Check sheet for the modelled part. Datum: model origin and axes. Units: mm. Coordinates: 2 decimals unless noted, no trailing zeros. Loops run counter-clockwise (first coordinate to the right, second up) from the corner with the lowest first, then second, coordinate; pieces in that order, holes last.
from build123d import *

# Parameters (mm, degrees)
SKETCH_R              = 23
SKETCH_R_2            = 2.75
SKETCH_R_3            = 2
PAD_DEPTH             = 1
SKETCH001_R           = 1.65
POCKET_DEPTH          = 1415.215977
POLARPATTERN_COUNT    = 3
POCKET001_DEPTH       = 5
SKETCH003_R           = 1.1
SKETCH003_R_2         = 1.45
POCKET002_DEPTH       = 1.001
SKETCH004_R           = 1.45
POCKET003_DEPTH       = 1.001
SKETCH005_R           = 2.1
POCKET004_DEPTH       = 1.001
SKETCH006_R           = 1.65
POCKET005_DEPTH       = 1415.215977
POLARPATTERN001_COUNT = 4
FILLET_R              = 15
PAD001_DEPTH          = 1


with BuildPart() as part:
    # Sketch → Pad (new body)
    with BuildSketch(Plane.XY):
        Polygon((103.553391, 250), (-103.553391, 250), (-250, 103.553391), (-250, -103.553391), (-103.553391, -250), (103.553391, -250), (250, -103.553391), (250, 103.553391), align=None)
        Circle(SKETCH_R, mode=Mode.SUBTRACT)
        with Locations((150, 150)):
            Circle(SKETCH_R_2, mode=Mode.SUBTRACT)
        with Locations((-150, 150)):
            Circle(SKETCH_R_2, mode=Mode.SUBTRACT)
        with Locations((-150, -150)):
            Circle(SKETCH_R_2, mode=Mode.SUBTRACT)
        with Locations((150, -150)):
            Circle(SKETCH_R_2, mode=Mode.SUBTRACT)
        with Locations((28.284271, 28.284271)):
            Circle(SKETCH_R_3, mode=Mode.SUBTRACT)
        with Locations((-28.284271, 28.284271)):
            Circle(SKETCH_R_3, mode=Mode.SUBTRACT)
        with Locations((-28.284271, -28.284271)):
            Circle(SKETCH_R_3, mode=Mode.SUBTRACT)
        with Locations((28.284271, -28.284271)):
            Circle(SKETCH_R_3, mode=Mode.SUBTRACT)
    extrude(amount=PAD_DEPTH)

    # Sketch001 → Pocket (cut, through all)
    with BuildSketch(Plane.XY):
        with Locations((169.926455, -5)):
            Circle(SKETCH001_R)
        with Locations((169.926455, -18)):
            Circle(SKETCH001_R)
    pocket = extrude(amount=POCKET_DEPTH, mode=Mode.SUBTRACT)

    # PolarPattern: Pocket ×3 about axis
    polarpattern_axis = Axis((0, 0, 0), (0, 0, 1))
    for i in range(1, POLARPATTERN_COUNT):
        add(pocket.rotate(polarpattern_axis, i * 360 / POLARPATTERN_COUNT), mode=Mode.SUBTRACT)

    # Sketch002 → Pocket001 (cut)
    with BuildSketch(Plane.XY):
        with BuildLine():
            ThreePointArc((-60, 8), (-68, 0), (-60, -8))
            Line((-60, -8), (60, -8))
            ThreePointArc((60, -8), (68, 0), (60, 8))
            Line((-60, 8), (60, 8))
        make_face()
    extrude(amount=POCKET001_DEPTH, mode=Mode.SUBTRACT)

    # Sketch003 → Pocket002 (cut, through all)
    with BuildSketch(Plane.XY):
        with Locations((-80, 71)):
            Circle(SKETCH003_R)
        with Locations((-80, 26)):
            Circle(SKETCH003_R)
        with Locations((-80, -26)):
            Circle(SKETCH003_R)
        with Locations((-80, -71)):
            Circle(SKETCH003_R)
        with Locations((-80, 0)):
            Circle(SKETCH003_R_2)
        with Locations((80, 71)):
            Circle(SKETCH003_R)
        with Locations((80, 26)):
            Circle(SKETCH003_R)
        with Locations((80, 0)):
            Circle(SKETCH003_R_2)
        with Locations((80, -26)):
            Circle(SKETCH003_R)
        with Locations((80, -71)):
            Circle(SKETCH003_R)
        Polygon((-95, 51), (-105, 51), (-105, 45), (-103.5, 45), (-103.5, 49.5), (-95, 49.5), align=None)
        Polygon((-105, -45), (-95, -45), (-101.312029, -49.5), (-96, -49.5), (-96, -51), (-106, -51), (-99.687971, -46.5), (-105, -46.5), align=None)
        Polygon((105, -51), (95, -51), (101.312029, -46.5), (96, -46.5), (96, -45), (106, -45), (99.687971, -49.5), (105, -49.5), align=None)
        Polygon((95, 45), (105, 45), (105, 51), (103.5, 51), (103.5, 46.5), (95, 46.5), align=None)
    extrude(amount=POCKET002_DEPTH, mode=Mode.SUBTRACT)

    # Sketch004 → Pocket003 (cut, through all)
    with BuildSketch(Plane.XY):
        with Locations((-32.5, -56.291651)):
            Circle(SKETCH004_R)
        with Locations((32.5, -56.291651)):
            Circle(SKETCH004_R)
        with Locations((-32.5, 56.291651)):
            Circle(SKETCH004_R)
        with Locations((32.5, 56.291651)):
            Circle(SKETCH004_R)
    extrude(amount=POCKET003_DEPTH, mode=Mode.SUBTRACT)

    # Sketch005 → Pocket004 (cut, through all)
    with BuildSketch(Plane.XY):
        with Locations((135, 150)):
            Circle(SKETCH005_R)
        with Locations((165, 150)):
            Circle(SKETCH005_R)
        with Locations((-165, 150)):
            Circle(SKETCH005_R)
        with Locations((-135, 150)):
            Circle(SKETCH005_R)
        with Locations((-165, -150)):
            Circle(SKETCH005_R)
        with Locations((-135, -150)):
            Circle(SKETCH005_R)
        with Locations((135, -150)):
            Circle(SKETCH005_R)
        with Locations((165, -150)):
            Circle(SKETCH005_R)
    extrude(amount=POCKET004_DEPTH, mode=Mode.SUBTRACT)

    # Sketch006 → Pocket005 (cut, through all)
    with BuildSketch(Plane.XY):
        with Locations((-161.970876, -52.035422)):
            Circle(SKETCH006_R)
        with Locations((-157.524615, -64.251426)):
            Circle(SKETCH006_R)
    pocket005 = extrude(amount=POCKET005_DEPTH, mode=Mode.SUBTRACT)

    # PolarPattern001: Pocket005 ×4 about axis
    polarpattern001_axis = Axis((0, 0, 0), (0, 0, 1))
    for i in range(1, POLARPATTERN001_COUNT):
        add(pocket005.rotate(polarpattern001_axis, i * 360 / POLARPATTERN001_COUNT), mode=Mode.SUBTRACT)

    # Fillet
    fillet_edges = [part.edges().sort_by_distance(p)[0] for p in [
        (-250, -103.553391, 0.5),
        (-103.553391, -250, 0.5),
        (103.553391, -250, 0.5),
        (-250, 103.553391, 0.5),
        (-103.553391, 250, 0.5),
        (103.553391, 250, 0.5),
        (250, 103.553391, 0.5),
        (250, -103.553391, 0.5),
    ]]
    fillet(fillet_edges, radius=FILLET_R)

    # Sketch007 → Pad001 (join)
    with BuildSketch(Plane.XY):
        Polygon((369.551813, 153.073373), (153.073373, 369.551813), (-153.073373, 369.551813), (-369.551813, 153.073373), (-369.551813, -153.073373), (-153.073373, -369.551813), (153.073373, -369.551813), (369.551813, -153.073373), align=None)
        Polygon((241.421356, 100), (100, 241.421356), (-100, 241.421356), (-241.421356, 100), (-241.421356, -100), (-100, -241.421356), (100, -241.421356), (241.421356, -100), align=None, mode=Mode.SUBTRACT)
    extrude(amount=PAD001_DEPTH)


solid = part.part
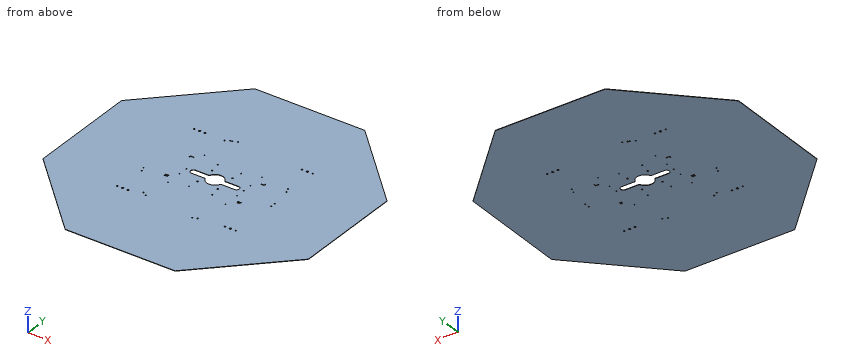
(1) Section check A-A, the plane z = 0.45. Count the separate pieces of the cut face and the enclosed holes in it, plus the area to 3 significant figures.
(2) Scan lines: line 1 along Y through (x, z) = (28, 0.95); line 2 along Y through (x, z) = (80, 0.3); line 3 along X through (y, z) = (-49, 0.95). Record each from-to range of solid material in increasing order.
(3) Section check B-B, the plane x = -258. Enter the section's corners in (y, z).
(4) Section check C-C, the plane y = 301. Enter the section's corners in (x, z).
Determined:
1. separate pieces: 1
1. enclosed holes: 49
1. area: 449,000 mm2
2. line 1: y = -369.55 to -30.26, -26.3 to -8, 8 to 26.3, 30.26 to 369.55
2. line 2: y = -369.55 to -72.1, -69.9 to -27.1, -24.9 to -1.45, 1.45 to 24.9, 27.1 to 69.9, 72.1 to 369.55
2. line 3: x = -369.55 to -103.19, -100.61 to 97.81, 100.39 to 369.55
3. outline: (-264.63, 0) - (264.63, 0) - (264.63, 1) - (-264.63, 1) - close
4. outline: (-221.63, 0) - (221.63, 0) - (221.63, 1) - (-221.63, 1) - close
